```python
from build123d import *

# Parameters (mm, degrees)
SKETCH_1_W          = 41
SKETCH_1_H          = 31
EXTRUDE_1_DEPTH     = 3.5
SKETCH_2_W          = 3.5
SKETCH_2_H          = 31
EXTRUDE_2_DEPTH     = 40
SKETCH_3_R          = 5.25
CUT_EXTRUDE_2_DEPTH = 62.753542409
SKETCH_4_R          = 3
CUT_EXTRUDE_3_DEPTH = 40


with BuildPart() as part:
    # 草图1 → 凸台-拉伸1 (new body)
    with BuildSketch(Plane(origin=(0, 0, 0), x_dir=(1, 0, 0), z_dir=(0, 1, 0))):
        Rectangle(SKETCH_1_W, SKETCH_1_H)
    extrude(amount=EXTRUDE_1_DEPTH)

    # 草图2 → 凸台-拉伸2 (add)
    with BuildSketch(Plane(origin=(0, 3.5, 0), x_dir=(1, 0, 0), z_dir=(0, 1, 0))):
        with Locations((-18.75, 0)):
            Rectangle(SKETCH_2_W, SKETCH_2_H)
        with Locations((18.75, 0)):
            Rectangle(SKETCH_2_W, SKETCH_2_H)
    extrude(amount=EXTRUDE_2_DEPTH)

    # 草图3 → 切除-拉伸2 (cut, through all)
    with BuildSketch(Plane(origin=(20.5, 0, 0), x_dir=(0, 0, -1), z_dir=(1, 0, 0))):
        with Locations((7.5, 26)):
            Circle(SKETCH_3_R)
        with BuildLine():
            Line((1.60695917, 31.41036688), (-15.5, 12.77724807))
            Line((-15.5, 12.77724807), (-15.5, 43.5))
            Line((-15.5, 43.5), (15.5, 43.5))
            Line((15.5, 43.5), (15.5, 26))
            ThreePointArc((15.5, 26), (10.403073661, 33.454673925), (1.60695917, 31.41036688))
        make_face()
    extrude(amount=-CUT_EXTRUDE_2_DEPTH, mode=Mode.SUBTRACT)

    # 草图4 → 切除-拉伸3 (cut)
    with BuildSketch(Plane(origin=(0, 3.5, 0), x_dir=(1, 0, 0), z_dir=(0, 1, 0))):
        with Locations(Location((0, -5.5, 0), (0, 0, 270))):
            Circle(SKETCH_4_R)
        with BuildLine():
            Line((-3, 10), (-3, 15.5))
            Line((-3, 15.5), (3, 15.5))
            Line((3, 15.5), (3, 10))
            ThreePointArc((3, 10), (0, 7), (-3, 10))
        make_face()
    extrude(amount=-CUT_EXTRUDE_3_DEPTH, mode=Mode.SUBTRACT)


solid = part.part
```
Source: CAD feature listing. Evaluate the final solid. Frame: model axes, mm. A direction names the side the tool comes from. Round coordinates to 2 decimals unless told otherwise and drop trailing zeros. Write each loop counter-clockwise with the first axis right and the second up, starting at its lowest first coordinate (ties: lowest second). Pieces come first, ordered by that corner, then holes. Notation, with made-up numbers: M 11,-23.75 L 36,-23.75 A27 cw 36,-7.75 Z; hole C 83.5,-18 d9. An arc over 180 degrees is marked long. Use CSV: the item, a comma, the result in double quotes. Start each with the question number.
Q1. Access query for faces 1 (the face through (-3, 2, -13)), 2 (the face through (17, 15, -3)), 3 (the face through (-18, 10, -15.5)). Directions: +Z, -Z, +X, -X, +Y, -Y. A direction counts if a zero-diameter tool reaches every point of the face in a straight line with its end or side. Return the directions, or none.
Q2. Line query: line 1 (X direction, y = 15, z = 5.5); line 2 (X direction, y = 3, z = -14); line 3 (Y direction, x = 15.5, z = 11.5). Output: solid intervals per line, ascending. Write a range as from..to.
Q3. Cut plane C-C on z = 8. Output: boundary loops of the cut face in (x, y), plus the area to 3 significant figures.
Q4. Pull-direction query (Z, two-part tool) for faces 4 (the face through (0, 2, -7)), 5 (the face through (18.77, 22.22, 6.83)), 6 (the face through (18.77, 21.34, -9.92)), 7 (the face through (-18.73, 21.34, -9.92)); classes: +Z half, -Z half, draft (parallel to the pull), parting line (faces both ways), or undercut.
Q5. Cut plane D-D on y = 24. Output: boundary loops of the cut face in (x, z).
Q6. Cut plane B-B on y = 7. Output: boundary loops of the cut face in (x, z).
Q7. Cut plane A-A on x = 0. Output: boundary loops of the cut face in (y, z), plus the area to 4 significant figures.
Q8. First-contact query: P1, Ø2, axis at x = 10, z = 8, coming from the +Y side. Flat tip, straight axial feed; report the tip coordinate or a pass-through.
Results found:
1,face 1,"-Z, +Y, -Y"
1,face 2,"+Z, -Z, +Y"
1,face 3,"-Z, +X, -X, +Y, -Y"
2,line 1,"-20.5..-17, 17..20.5"
2,line 2,"-20.5..-3, 3..20.5"
2,line 3,"0..3.5"
3,outline,"M -20.5,0 L -1.66,0 L -1.66,3.5 L -17,3.5 L -17,20.95 L -20.5,20.95 Z; M 1.66,0 L 20.5,0 L 20.5,20.95 L 17,20.95 L 17,3.5 L 1.66,3.5 Z"
3,area,"254 mm^2"
4,face 4,"-Z half"
4,face 5,"+Z half"
4,face 6,"undercut"
4,face 7,"undercut"
5,outline,"M -20.5,-15.5 L -17,-15.5 L -17,-12.35 L -20.5,-12.35 Z; M -20.5,-2.65 L -17,-2.65 L -17,5.2 L -20.5,5.2 Z; M 17,-15.5 L 20.5,-15.5 L 20.5,-12.35 L 17,-12.35 Z; M 17,-2.65 L 20.5,-2.65 L 20.5,5.2 L 17,5.2 Z"
6,outline,"M -20.5,-15.5 L -17,-15.5 L -17,15.5 L -20.5,15.5 Z; M 17,-15.5 L 20.5,-15.5 L 20.5,15.5 L 17,15.5 Z"
7,outline,"M 0,-7 L 3.5,-7 L 3.5,2.5 L 0,2.5 Z; M 0,8.5 L 3.5,8.5 L 3.5,15.5 L 0,15.5 Z"
7,area,"57.75 mm^2"
8,P1,"y = 3.5"
